Verification items for the finished model (mm, model axes). Face numbers are marked on the shaded views. A direction names the side the tool comes from. Coordinates: 2 decimals unless noted, no trailing zeros. Order: outer loops, then holes, each group sorted by start corner. A loop starts at its lowest first (then second) coordinate and runs counter-clockwise, first axis right, second up. Notation, with made-up numbers: (10, 36) -> (64, 36) arc R24 cw to (64, 59) -> close; hole circle Ø4 at (24.25, 63). An arc over 180 degrees is marked (long way). Write each question's results on one line, items separated by ' | '. Start each with the question number.
(1) Cross-section at D-D on x = -98.5. Enter the section's corners in (y, z).
(2) Cross-section at C-C on x = 276.5. Enter the section's corners in (y, z).
(3) Thickness scan on probe 1 along Z at (x, y) = (-136, 217.5); probe 2 along X at (y, z) = (35, 721); probe 3 along Z at (x, y) = (-277.5, 39.5). Record the ranges inside material, lowest first. Write a range as [from, to].
(4) Cross-section at A-A on z = 376.5. Enter the section's corners in (x, y).
(5) Set-up check for the marked faces 1 and 2: record each of +Z, -Z, +X, -X, +Y, -Y from which the full face is reachable in a straight line by a thin tool's end or side.
(6) Cross-section at B-B on y = 110. Enter the section's corners in (x, z), and give its area (3 significant figures).
```python
from build123d import *

# Parameters (mm, degrees)
CROQUIS1_W               = 950
CROQUIS1_H               = 2000
CROQUIS1_W_2             = 900
CROQUIS1_H_2             = 1950
SALIENTE_EXTRUIR1_DEPTH  = 50
CROQUIS3_W               = 950
CROQUIS3_H               = 50
SALIENTE_EXTRUIR3_DEPTH  = 50
CROQUIS6_W               = 950
CROQUIS6_H               = 50
SALIENTE_EXTRUIR6_DEPTH  = 50
CROQUIS4_W               = 950
CROQUIS4_H               = 50
SALIENTE_EXTRUIR7_DEPTH  = 400
SALIENTE_EXTRUIR8_DEPTH  = 50
CROQUIS9_W               = 950
CROQUIS9_H               = 50
SALIENTE_EXTRUIR9_DEPTH  = 300
SALIENTE_EXTRUIR10_DEPTH = 50


with BuildPart() as part:
    # Croquis1 → Saliente-Extruir1 (new body)
    with BuildSketch(Plane(origin=(0, 0, 0), x_dir=(1, 0, 0), z_dir=(0, 1, 0))):
        Rectangle(CROQUIS1_W, CROQUIS1_H)
        Rectangle(CROQUIS1_W_2, CROQUIS1_H_2, mode=Mode.SUBTRACT)
    extrude(amount=SALIENTE_EXTRUIR1_DEPTH)

    # Croquis3 → Saliente-Extruir3 (add)
    with BuildSketch(Plane(origin=(0, 0, -1000), x_dir=(-1, 0, 0), z_dir=(0, 0, -1))):
        with Locations((0, 25)):
            Rectangle(CROQUIS3_W, CROQUIS3_H)
    extrude(amount=SALIENTE_EXTRUIR3_DEPTH)

    # Croquis6 → Saliente-Extruir6 (add)
    with BuildSketch(Plane.XY.offset(1000)):
        with Locations((0, 25)):
            Rectangle(CROQUIS6_W, CROQUIS6_H)
    extrude(amount=SALIENTE_EXTRUIR6_DEPTH)

    # Croquis4 → Saliente-Extruir7 (add)
    with BuildSketch(Plane(origin=(0, 50, 0), x_dir=(1, 0, 0), z_dir=(0, 1, 0))):
        with Locations((0, 1025)):
            Rectangle(CROQUIS4_W, CROQUIS4_H)
    extrude(amount=SALIENTE_EXTRUIR7_DEPTH)

    # Croquis8 → Saliente-Extruir8 (add)
    with BuildSketch(Plane(origin=(0, 0, -1050), x_dir=(-1, 0, 0), z_dir=(0, 0, -1))):
        with BuildLine():
            Line((-475, 450), (475, 450))
            ThreePointArc((475, 450), (0, 550.017484419), (-475, 450))
        make_face()
    extrude(amount=-SALIENTE_EXTRUIR8_DEPTH)

    # Croquis9 → Saliente-Extruir9 (add)
    with BuildSketch(Plane(origin=(0, 50, 0), x_dir=(1, 0, 0), z_dir=(0, 1, 0))):
        with Locations((0, -1025)):
            Rectangle(CROQUIS9_W, CROQUIS9_H)
    extrude(amount=SALIENTE_EXTRUIR9_DEPTH)

    # Croquis10 → Saliente-Extruir10 (add)
    with BuildSketch(Plane.XY.offset(1050)):
        with BuildLine():
            Line((-475, 350), (475, 350))
            ThreePointArc((475, 350), (0, 449.957514301), (-475, 350))
        make_face()
    extrude(amount=-SALIENTE_EXTRUIR10_DEPTH)


solid = part.part
```
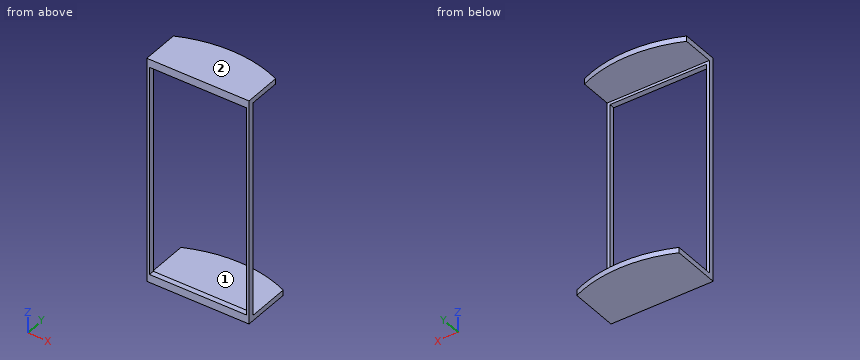
Results are:
1) outline: (0, -1050) -> (545.89, -1050) -> (545.89, -1000) -> (50, -1000) -> (50, -975) -> (0, -975) -> close; (0, 975) -> (50, 975) -> (50, 1000) -> (445.83, 1000) -> (445.83, 1050) -> (0, 1050) -> close
2) outline: (0, -1050) -> (517.11, -1050) -> (517.11, -1000) -> (50, -1000) -> (50, -975) -> (0, -975) -> close; (0, 975) -> (50, 975) -> (50, 1000) -> (417.06, 1000) -> (417.06, 1050) -> (0, 1050) -> close
3) probe 1: z = [-1050, -1000], [1000, 1050] | probe 2: x = [-475, -450], [450, 475] | probe 3: z = [-1050, -975], [975, 1050]
4) outline: (-475, 0) -> (-450, 0) -> (-450, 50) -> (-475, 50) -> close; (450, 0) -> (475, 0) -> (475, 50) -> (450, 50) -> close
5) face 1: +X, -X, +Y | face 2: +Z, +X, -X, +Y, -Y
6) outline: (-475, -1050) -> (475, -1050) -> (475, -1000) -> (-475, -1000) -> close; (-475, 1000) -> (475, 1000) -> (475, 1050) -> (-475, 1050) -> close | area: 95,000 mm2
